Geometry check sheet. Reference: the model listing, model coordinates, mm. Give positions to 0.01 mm unless a question says otherwise; leave off trailing zeros. Loops run counter-clockwise (first coordinate to the right, second up) from the corner with the lowest first, then second, coordinate; pieces in that order, holes last.
1. Cross-section at A-A, the plane x = -12.5. Record the cut outline in (y, z).
2. Go/stop test with flat-tipped pins: pin 1 Ø1.2 at (x, y) = (51, 2) entering from +Z; pin 2 Ø3 at (x, z) = (-12.5, -16.5) entering from -Y; pin 3 Ø2 at (y, z) = (2.5, -23.5) entering from +X; pin 4 Ø2 at (y, z) = (0.5, 2) entering from +X. Record where each tip stops, or that it passes through.
3. Cross-section at D-D, the plane y = 1.2. State how many separate pieces and enclosed holes the cut face has, plus the area to 3 significant figures.
4. Release check for a two-part mould opening along X. For faces 1 (the flat face through (0, 2, -6.637)), 2 (the flat face through (0, 2, 10)), 3 (the flat face through (-25, 2, 5)) record: +X half, -X half, draft (parallel to the pull), parting line (faces both ways), or undercut.
5. Cross-section at B-B, the plane x = -56.5. Record the cut outline in (y, z).
6. Cross-section at C-C, the plane z = -44.5. Record the cut outline in (x, y).
7. Material ranges on L1, parallel to Z at x = -20, y = 2.6 (3 decimals); L2, parallel to X at y = 1.95, z = -20; L3, parallel to X at y = 2.55, z = -25, recorded low to high.
from build123d import *

# Parameters (mm, degrees)
EXTRUDE_1_DEPTH     = 4
SKETCH_2_R          = 1.6
CUT_EXTRUDE_1_DEPTH = 100.483667001
SKETCH_4_R          = 1.275
CUT_EXTRUDE_3_DEPTH = 10
SKETCH_6_W          = 50
SKETCH_6_H          = 10
EXTRUDE_2_DEPTH     = 4
SKETCH_7_R          = 2.1
CUT_EXTRUDE_4_DEPTH = 10
SKETCH_8_R          = 2
CUT_EXTRUDE_5_DEPTH = 10
CUT_EXTRUDE_6_DEPTH = 10
CUT_EXTRUDE_7_DEPTH = 10
FILLET_2_R          = 2


with BuildPart() as part:
    # 草图1 → 凸台-拉伸1 (new body)
    with BuildSketch(Plane(origin=(0, 0, 0), x_dir=(1, 0, 0), z_dir=(0, 1, 0))):
        Polygon((25, 0), (-25, 0), (-80, 29), (-80, 59), (80, 59), (80, 29), align=None)
    extrude(amount=EXTRUDE_1_DEPTH)

    # 草图2 → 切除-拉伸1 (cut, through all)
    with BuildSketch(Plane(origin=(0, 4, 0), x_dir=(1, 0, 0), z_dir=(0, 1, 0))):
        with Locations(Location((-12.5, 41.5, 0), (0, 0, 270))):
            Circle(SKETCH_2_R)
        with Locations(Location((12.5, 41.5, 0), (0, 0, 90))):
            Circle(SKETCH_2_R)
        with Locations(Location((-12.5, 16.5, 0), (0, 0, 90))):
            Circle(SKETCH_2_R)
        with Locations(Location((12.5, 16.5, 0), (0, 0, 270))):
            Circle(SKETCH_2_R)
    extrude(amount=-CUT_EXTRUDE_1_DEPTH, mode=Mode.SUBTRACT)

    # 草图4 → 切除-拉伸3 (cut)
    with BuildSketch(Plane(origin=(0, 4, 0), x_dir=(1, 0, 0), z_dir=(0, 1, 0))):
        with Locations(Location((20, 50, 0), (0, 0, 270))):
            Circle(SKETCH_4_R)
        with Locations(Location((20, 30, 0), (0, 0, 270))):
            Circle(SKETCH_4_R)
        with Locations(Location((-20, 30, 0), (0, 0, 90))):
            Circle(SKETCH_4_R)
        with Locations(Location((-20, 50, 0), (0, 0, 90))):
            Circle(SKETCH_4_R)
    extrude(amount=-CUT_EXTRUDE_3_DEPTH, mode=Mode.SUBTRACT)

    # 草图6 → 凸台-拉伸2 (add)
    with BuildSketch(Plane(origin=(0, 4, 0), x_dir=(1, 0, 0), z_dir=(0, 1, 0))):
        with Locations((0, -5)):
            Rectangle(SKETCH_6_W, SKETCH_6_H)
    extrude(amount=-EXTRUDE_2_DEPTH)

    # 草图7 → 切除-拉伸4 (cut)
    with BuildSketch(Plane(origin=(0, 4, 0), x_dir=(1, 0, 0), z_dir=(0, 1, 0))):
        with Locations(Location((-6, -6, 0), (0, 0, 270))):
            Circle(SKETCH_7_R)
        with Locations(Location((6, -6, 0), (0, 0, 90))):
            Circle(SKETCH_7_R)
    extrude(amount=-CUT_EXTRUDE_4_DEPTH, mode=Mode.SUBTRACT)

    # 草图8 → 切除-拉伸5 (cut)
    with BuildSketch(Plane(origin=(0, 4, 0), x_dir=(1, 0, 0), z_dir=(0, 1, 0))):
        with Locations(Location((-73, 49, 0), (0, 0, 270))):
            Circle(SKETCH_8_R)
        with Locations(Location((73, 49, 0), (0, 0, 90))):
            Circle(SKETCH_8_R)
    extrude(amount=-CUT_EXTRUDE_5_DEPTH, mode=Mode.SUBTRACT)

    # 草图9 → 切除-拉伸6 (cut)
    with BuildSketch(Plane(origin=(0, 4, 0), x_dir=(1, 0, 0), z_dir=(0, 1, 0))):
        Polygon((-13.607153835, 27.875584016), (13.607153835, 27.875584016), (0, 21.424785161), align=None)
        Polygon((-61.511227824, 51), (-33.511227824, 51), (-60.564799252, 38.03449681), align=None)
        Polygon((-51.708784474, 24.598987773), (-29.079791665, 35.443998725), (-29.079791665, 12.667337019), align=None)
        Polygon((29.079791665, 12.667337019), (51.708784474, 24.598987773), (29.079791665, 35.443998725), align=None)
        Polygon((60.564799252, 38.03449681), (61.511227824, 51), (33.511227824, 51), align=None)
    extrude(amount=-CUT_EXTRUDE_6_DEPTH, mode=Mode.SUBTRACT)

    # 草图10 → 切除-拉伸7 (cut)
    with BuildSketch(Plane(origin=(0, 4, 0), x_dir=(1, 0, 0), z_dir=(0, 1, 0))):
        Polygon((-15.862821337, 6.636596525), (15.862821337, 6.636596525), (0, -1.727436544), align=None)
    extrude(amount=-CUT_EXTRUDE_7_DEPTH, mode=Mode.SUBTRACT)

    # 圆角2
    fillet_2_edges = [part.edges().sort_by_distance(p)[0] for p in [
        (25, 2, 0),
        (-25, 2, 0),
        (60.564799252, 2, -38.03449681),
        (33.511227824, 2, -51),
        (61.511227824, 2, -51),
        (29.079791665, 2, -12.667337019),
        (29.079791665, 2, -35.443998725),
        (51.708784474, 2, -24.598987773),
        (-29.079791665, 2, -12.667337019),
        (-51.708784474, 2, -24.598987773),
        (-29.079791665, 2, -35.443998725),
        (-60.564799252, 2, -38.03449681),
        (-61.511227824, 2, -51),
        (-33.511227824, 2, -51),
        (0, 2, -21.424785161),
        (-13.607153835, 2, -27.875584016),
        (13.607153835, 2, -27.875584016),
        (15.862821337, 2, -6.636596525),
        (0, 2, 1.727436544),
        (-15.862821337, 2, -6.636596525),
        (25, 2, 10),
        (-25, 2, 10),
    ]]
    fillet(fillet_2_edges, radius=FILLET_2_R)


solid = part.part
Result:
1. outline: (0, -59) - (4, -59) - (4, -43.1) - (0, -43.1) - close; (0, -39.9) - (4, -39.9) - (4, -18.1) - (0, -18.1) - close; (0, -14.9) - (4, -14.9) - (4, 10) - (0, 10) - close
2. pin 1: stops at z = -13.39
2. pin 2: passes through
2. pin 3: stops at x = 71.47
2. pin 4: stops at x = 25.01
3. separate pieces: 1
3. enclosed holes: 18
3. area: 7,230 mm2
4. face 1: undercut
4. face 2: draft
4. face 3: -X half
5. outline: (0, -59) - (4, -59) - (4, -51) - (0, -51) - close; (0, -39.98) - (4, -39.98) - (4, -16.61) - (0, -16.61) - close
6. outline: (-80, 0) - (-61.04, 0) - (-61.04, 4) - (-80, 4) - close; (-47.07, 0) - (47.07, 0) - (47.07, 4) - (-47.07, 4) - close; (61.04, 0) - (80, 0) - (80, 4) - (61.04, 4) - close
7. L1: z = -59 to -51.275, -48.725 to -31.275, -28.725 to 10
7. L2: x = -62.93 to -42.99, -29.08 to 29.08, 42.99 to 62.93
7. L3: x = -72.41 to -49.2, -29.08 to -6.52, 6.52 to 29.08, 49.2 to 72.41
